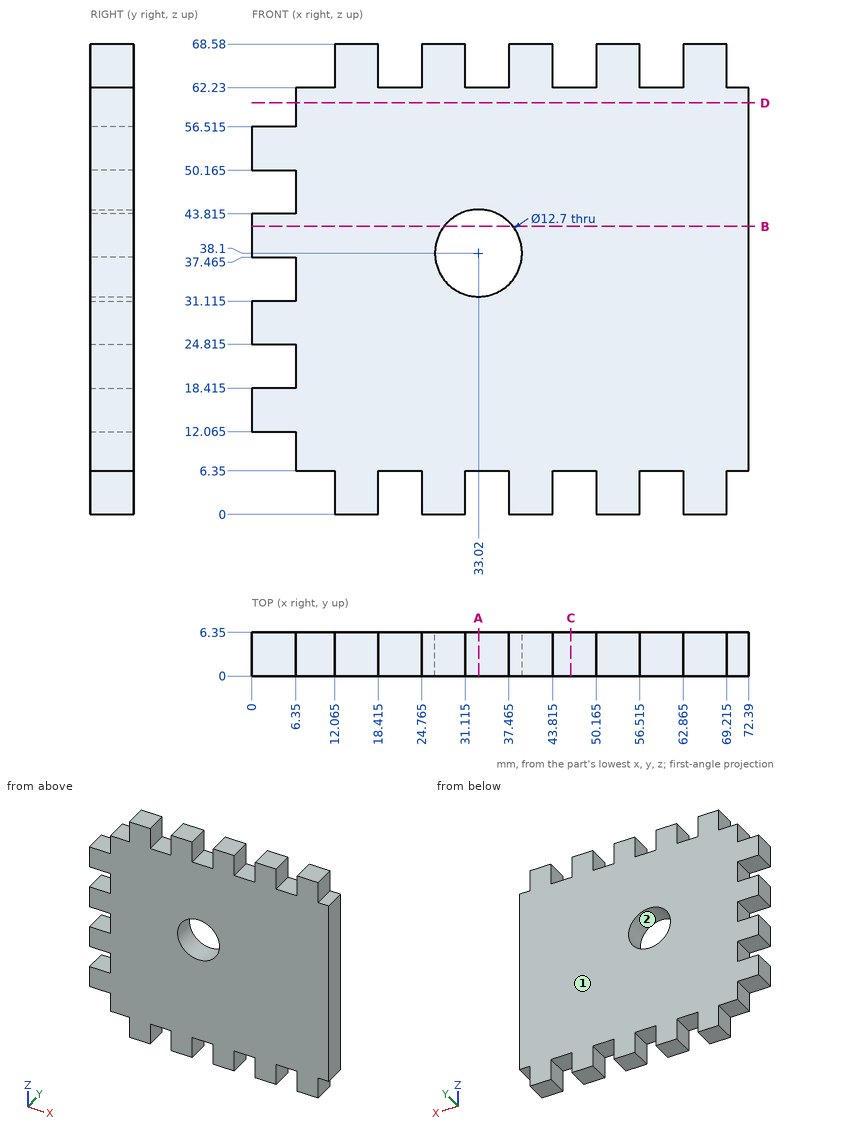
Input: dimensioned drawing with shaded views. Units: mm. Origin: part minimum x, y, z. Round coordinates to 2 decimals unless told otherwise and drop trailing zeros. Loops run counter-clockwise (first coordinate to the right, second up) from the corner with the lowest first, then second, coordinate; pieces in that order, holes last. Notation, with made-up numbers: M 47,31 L 101,31 A23 ccw 101,60 Z; hole C 19.5,75.5 d5. An arc over 180 degrees is marked long. Answer in a Markdown table with one row per item. Add a question column.
1. Section D-D (z = 60). Output: boundary loops of the cut face in (x, y), and give its area (3 significant figures).
2. Contact query for flat-ended pins moving along their axis: pin 1 (4 mm diameter, centred on x = 24, z = 45.5, fed in from -Y); pin 2 (3 mm diameter, centred on y = 4, z = 4, fed in from +X) (3 decimals); pin 3 (1.9 mm diameter, centred on x = 3, y = 3, fed in from +Z) (3 decimals); pin 4 (1.9 mm diameter, centred on x = 33.5, y = 2.5, fed in from -Z). Output: stop coordinate, or through.
3. Section C-C (x = 46.5). Output: boundary loops of the cut face in (y, z), and give its area (3 significant figures).
4. Section B-B (z = 42). Output: boundary loops of the cut face in (x, y), and give its area (3 significant figures).
5. Mould query, pull axis Z, two halves, no side actions, for the marked faces 1 and 2. Classes: released by +Z, released by -Z, zero draft, split by the parting line, or undercut.
6. Section A-A (x = 33.02). Output: boundary loops of the cut face in (y, z), and give its area (3 significant figures).
7. Ray query, probe 1 along X at (y, z) = (1.5, 62.5) (3 decimals); probe 2 along Z at (x, y) = (33.02, 1.5); probe 3 along X at (y, z) = (5.75, 50). Return the intervals inside material, ascending.
Values follow:
| question | item | result |
|---|---|---|
| 1 | outline | M 6.35,0 L 72.39,0 L 72.39,6.35 L 6.35,6.35 Z |
| 1 | area | 419 mm^2 |
| 2 | pin 1 | y = 0 |
| 2 | pin 2 | x = 69.215 |
| 2 | pin 3 | z = 56.515 |
| 2 | pin 4 | z = 6.35 |
| 3 | outline | M 0,6.35 L 6.35,6.35 L 6.35,62.23 L 0,62.23 Z |
| 3 | area | 355 mm^2 |
| 4 | outline | M 0,0 L 28.01,0 L 28.01,6.35 L 0,6.35 Z; M 38.03,0 L 72.39,0 L 72.39,6.35 L 38.03,6.35 Z |
| 4 | area | 396 mm^2 |
| 5 | face 1 | zero draft |
| 5 | face 2 | undercut |
| 6 | outline | M 0,6.35 L 6.35,6.35 L 6.35,31.75 L 0,31.75 Z; M 0,44.45 L 6.35,44.45 L 6.35,62.23 L 0,62.23 Z |
| 6 | area | 274 mm^2 |
| 7 | probe 1 | 12.065 to 18.415, 24.765 to 31.115, 37.465 to 43.815, 50.165 to 56.515, 62.865 to 69.215 |
| 7 | probe 2 | 6.35 to 31.75, 44.45 to 62.23 |
| 7 | probe 3 | 6.35 to 72.39 |
